```python
from build123d import *

# Parameters (mm, degrees)
ESQUISSE1_R                  = 11
BOSS_EXTRU_1_DEPTH           = 5
ESQUISSE2_R                  = 9
BOSS_EXTRU_2_DEPTH           = 8
ESQUISSE3_R                  = 14
BOSS_EXTRU_3_DEPTH           = 6.35
ESQUISSE4_R                  = 7.5
BOSS_EXTRU_5_DEPTH           = 7
ENL_V_MAT_EXTRU_1_DEPTH      = 28.684336727
ENL_V_MAT_EXTRU_1_DEPTH_BACK = 28.684336727
ESQUISSE5_R                  = 1.25
ESQUISSE6_R                  = 6.5
ENL_V_MAT_EXTRU_2_DEPTH      = 13
CONG_3_R                     = 2


with BuildPart() as part:
    # Esquisse1 → Boss.-Extru.1 (new body)
    with BuildSketch(Plane(origin=(0, 0, 0), x_dir=(1, 0, 0), z_dir=(0, 1, 0))):
        with Locations(Location((0, 0, 0), (0, 0, 270))):
            Circle(ESQUISSE1_R)
    extrude(amount=BOSS_EXTRU_1_DEPTH)

    # Esquisse2 → Boss.-Extru.2 (add)
    with BuildSketch(Plane(origin=(0, 5, 0), x_dir=(1, 0, 0), z_dir=(0, 1, 0))):
        with Locations(Location((0, 0, 0), (0, 0, 270))):
            Circle(ESQUISSE2_R)
    extrude(amount=BOSS_EXTRU_2_DEPTH)

    # Esquisse3 → Boss.-Extru.3 (add)
    with BuildSketch(Plane.XZ):
        with Locations(Location((0, 0, 0), (0, 0, 270))):
            Circle(ESQUISSE3_R)
    extrude(amount=BOSS_EXTRU_3_DEPTH)

    # Esquisse4 → Boss.-Extru.5 (add)
    with BuildSketch(Plane.XZ.offset(6.35)):
        with Locations(Location((0, 0, 0), (0, 0, 270))):
            Circle(ESQUISSE4_R)
        with BuildLine():
            Line((1.775, -2.034545404), (1.775, 2.034545404))
            ThreePointArc((1.775, 2.034545404), (0, 2.7), (-1.775, 2.034545404))
            Line((-1.775, 2.034545404), (-1.775, -2.034545404))
            ThreePointArc((-1.775, -2.034545404), (0, -2.7), (1.775, -2.034545404))
        make_face(mode=Mode.SUBTRACT)
    extrude(amount=BOSS_EXTRU_5_DEPTH)

    # Esquisse5 → Enlèv. mat.-Extru.1 (cut, two sides: drawn at the far end of the back side and taken through both)
    with BuildSketch(Plane.XZ.offset(6.35).offset(-ENL_V_MAT_EXTRU_1_DEPTH_BACK)):
        with Locations(Location((0, 0, 0), (0, 0, 270))):
            Circle(ESQUISSE5_R)
    extrude(amount=ENL_V_MAT_EXTRU_1_DEPTH + ENL_V_MAT_EXTRU_1_DEPTH_BACK, mode=Mode.SUBTRACT)

    # Esquisse6 → Enlèv. mat.-Extru.2 (cut)
    with BuildSketch(Plane(origin=(0, 13, 0), x_dir=(1, 0, 0), z_dir=(0, 1, 0))):
        with Locations(Location((0, 0, 0), (0, 0, 270))):
            Circle(ESQUISSE6_R)
    extrude(amount=-ENL_V_MAT_EXTRU_2_DEPTH, mode=Mode.SUBTRACT)

    # Congé3
    cong_3_edges = [part.edges().sort_by_distance(p)[0] for p in [
        (0, -6.35, 7.5),
    ]]
    fillet(cong_3_edges, radius=CONG_3_R)


solid = part.part
```
Here's how the part is built. I have some questions about the finished solid (model axes, mm). A direction names the side the tool comes from. Coordinates: 2 decimals unless noted, no trailing zeros. Order: outer loops, then holes, each group sorted by start corner. A loop starts at its lowest first (then second) coordinate and runs counter-clockwise, first axis right, second up.
1) Which directions (+Z, -Z, +X, -X, +Y, -Y) give clear straight access to the entire face, cutting with the end or side of a thin tool? Please do faces 1 (the face through (-9.1, -6.35, 3.3)), 2 (the face through (-13.67, -3.13, 3.03)), 3 (the face through (2.703, 8.944, 8.584)).
2) Will these pins go through, and if not, where does the flat tip stop? pin 1 (8 mm diameter, centred on x = 0, z = 0, fed in from +Y); pin 2 (4 mm diameter, centred on y = -2.5, z = 10.5, fed in from -X); pin 3 (1 mm diameter, centred on y = -4.5, z = -11, fed in from -X).
3) Imagine slicing it at D-D on y = 9.25. List the corners of the cut face in (x, z) for me.
4) I need wall thicknesses on line 1 (X direction, y = 5.5, z = 0); line 2 (Z direction, x = -5, y = 9.5); line 3 (Y direction, x = 5.5, z = -0.75). Which ranges of each line are inside material? Lowest first, please.
5) We'd pull the mould along X, two halves only. Please class faces 4 (the face through (0.33, -10.815, 7.493)), 5 (the face through (0.1, 0, 1.4)), 6 (the face through (1.775, -10, 0)), 7 (the face through (-6, 13, 3)): +X half, -X half, draft (parallel to the pull), parting line (faces both ways), or undercut.
6) Imagine slicing it at C-C on y = -10.5. List the corners of the cut face in (x, z) for me (3 decimals), and give its area (3 significant figures).
Response values:
1. face 1: -Y
1. face 2: +Y, -Y
1. face 3: +Y
2. pin 1: stops at y = 0
2. pin 2: stops at x = -11.12
2. pin 3: stops at x = -9.26
3. outline: circle Ø18 at (0, 0); hole circle Ø13 at (0, 0)
4. line 1: x = -9 to -6.5, 6.5 to 9
4. line 2: z = -7.48 to -4.15, 4.15 to 7.48
4. line 3: y = -13.35 to 0
5. face 4: parting line
5. face 5: undercut
5. face 6: undercut
5. face 7: draft
6. outline: circle Ø15 at (0, 0); hole (-1.775, -2.035) arc R2.7 ccw to (1.775, -2.035) - (1.775, 2.035) arc R2.7 ccw to (-1.775, 2.035) - close
6. area: 159 mm2
